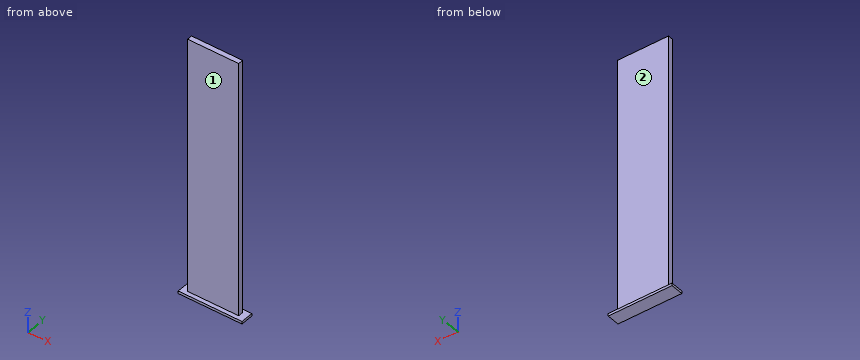
```python
from build123d import *

# Parameters (mm, degrees)
ESBO_O2_W                = 250
ESBO_O2_H                = 50
RESSALTO_EXTRUS_O1_DEPTH = 10
ESBO_O4_W                = 200
ESBO_O4_H                = 20
RESSALTO_EXTRUS_O2_DEPTH = 1000


with BuildPart() as part:
    # Esboço2 → Ressalto-extrusão1 (new body)
    with BuildSketch(Plane.XY):
        with Locations((125, 25)):
            Rectangle(ESBO_O2_W, ESBO_O2_H)
    extrude(amount=RESSALTO_EXTRUS_O1_DEPTH)

    # Esboço4 → Ressalto-extrusão2 (add)
    with BuildSketch(Plane.XY.offset(10)):
        with Locations((124.287859988, 26.407647707)):
            Rectangle(ESBO_O4_W, ESBO_O4_H)
    extrude(amount=RESSALTO_EXTRUS_O2_DEPTH)


solid = part.part
```
Read the model definition and answer for the solid it produces. Units are mm, in the model's axes. Face numbers are marked on the shaded views. A direction names the side the tool comes from. Round coordinates to 2 decimals unless told otherwise and drop trailing zeros. Loops run counter-clockwise (first coordinate to the right, second up) from the corner with the lowest first, then second, coordinate; pieces in that order, holes last. Notation, with made-up numbers: (-3, 76.5) -> (37, 76.5) arc R22 cw to (37, 95.5) -> close; hole circle Ø2 at (12.5, 86.25). An arc over 180 degrees is marked (long way). One line per item, written item: value.
1) For the marked faces 1 and 2, determine the directions among +Z, -Z, +X, -X, +Y, -Y from which every point of the face is accessible in a straight line to the end or side of a thin tool.
Answer list:
face 1: +Z, +X, -X, -Y
face 2: +Z, +X, -X, +Y
2) Flat-ended cylindrical pins translate along their axes: P1, Ø5, axis at x = 193.5, y = 26, coming from the -Z side; P2, Ø5, axis at x = 132, y = 10.5, coming from the +Z side; P3, Ø1.5, axis at x = 130.5, z = 807, coming from the -Y side; P4, Ø16, axis at y = 26, z = 265.5, coming from the +X side. Find the tip coordinate at first contact, or state that the pin passes through.
Answer list:
P1: stops at z = 0
P2: stops at z = 10
P3: stops at y = 16.41
P4: stops at x = 224.29
3) A cutting plane is placed at A-A (y = 26). Determine the outline of the cut face in (x, z).
Answer list:
outline: (0, 0) -> (250, 0) -> (250, 10) -> (224.29, 10) -> (224.29, 1010) -> (24.29, 1010) -> (24.29, 10) -> (0, 10) -> close
4) Consider L1, parallel to Y at x = 27.5, z = 326.5; L2, parallel to X at y = 17, z = 849; L3, parallel to Z at x = 100.5, y = 37.5. Determine where each line is inside the solid, lowest interval first. Write a range as [from, to].
Answer list:
L1: y = [16.41, 36.41]
L2: x = [24.29, 224.29]
L3: z = [0, 10]
5) A cutting plane is placed at C-C (z = 120). Determine the outline of the cut face in (x, y), and give its area (3 significant figures).
Answer list:
outline: (24.29, 16.41) -> (224.29, 16.41) -> (224.29, 36.41) -> (24.29, 36.41) -> close
area: 4,000 mm²
6) A cutting plane is placed at B-B (x = 126). Determine the outline of the cut face in (y, z), and give its area (3 significant figures).
Answer list:
outline: (0, 0) -> (50, 0) -> (50, 10) -> (36.41, 10) -> (36.41, 1010) -> (16.41, 1010) -> (16.41, 10) -> (0, 10) -> close
area: 20,500 mm²
